```python
from build123d import *

# Parameters (mm, degrees)
SKETCH1_W           = 311.15
SKETCH1_H           = 266.7
SKETCH1_W_2         = 295.275
SKETCH1_H_2         = 250.825
BOSS_EXTRUDE1_DEPTH = 20.6375
SKETCH2_R           = 2.54
CUT_EXTRUDE1_DEPTH  = 320.049014669
SKETCH3_R           = 2.54
CUT_EXTRUDE2_DEPTH  = 373.362542974


with BuildPart() as part:
    # Sketch1 → Boss-Extrude1 (new body)
    with BuildSketch(Plane(origin=(0, 0, 0), x_dir=(1, 0, 0), z_dir=(0, 1, 0))):
        with Locations((-18.31426751, -70.1534017)):
            Rectangle(SKETCH1_W, SKETCH1_H)
        with Locations((-18.31426751, -70.1534017)):
            Rectangle(SKETCH1_W_2, SKETCH1_H_2, mode=Mode.SUBTRACT)
    extrude(amount=BOSS_EXTRUDE1_DEPTH)

    # Sketch2 → Cut-Extrude1 (cut, through all)
    with BuildSketch(Plane.XY.offset(203.5034017)):
        with Locations((-18.31426751, 10.31875)):
            Circle(SKETCH2_R)
    extrude(amount=-CUT_EXTRUDE1_DEPTH, mode=Mode.SUBTRACT)

    # Sketch3 → Cut-Extrude2 (cut, through all)
    with BuildSketch(Plane(origin=(137.26073249, 0, 0), x_dir=(0, 0, -1), z_dir=(1, 0, 0))):
        with Locations((-70.1534017, 10.31875)):
            Circle(SKETCH3_R)
    extrude(amount=-CUT_EXTRUDE2_DEPTH, mode=Mode.SUBTRACT)


solid = part.part
```
Verification items for the finished model (mm, model axes). A direction names the side the tool comes from. Give positions to 0.01 mm unless a question says otherwise; leave off trailing zeros. Order: outer loops, then holes, each group sorted by start corner. A loop starts at its lowest first (then second) coordinate and runs counter-clockwise, first axis right, second up. Notation, with made-up numbers: (49, 15.25) -> (96, 15.25) arc R36 ccw to (96, 49.25) -> close; hole circle Ø2 at (69, 33). An arc over 180 degrees is marked (long way). Use a Markdown table: item, result.
1) Section check B-B, the plane z = 181.5. Record the boundary of the cut face in (x, y), then the cut area to 3 significant figures.
Results:
| item | result |
|---|---|
| outline | (-173.89, 0) -> (-165.95, 0) -> (-165.95, 20.64) -> (-173.89, 20.64) -> close; (129.32, 0) -> (137.26, 0) -> (137.26, 20.64) -> (129.32, 20.64) -> close |
| area | 328 mm² |
2) Section check A-A, the plane x = -72. Record the boundary of the cut face in (y, z), then the cut area to 3 significant figures.
Results:
| item | result |
|---|---|
| outline | (0, -63.2) -> (20.64, -63.2) -> (20.64, -55.26) -> (0, -55.26) -> close; (0, 195.57) -> (20.64, 195.57) -> (20.64, 203.5) -> (0, 203.5) -> close |
| area | 328 mm² |
3) Material ranges on probe 1 along X at (y, z) = (4.75, 80); probe 2 along Z at (x, y) = (-9.5, 5.75), recorded low to high.
Results:
| item | result |
|---|---|
| probe 1 | -173.89 to -165.95, 129.32 to 137.26 |
| probe 2 | -63.2 to -55.26, 195.57 to 203.5 |
4) Mould release check, pull along X, two halves, no side actions. Record for faces 1 (the flat face through (-165.952, 12.5, 71.9)), 2 (the flat face through (-20.5, 12.5, 203.503)), 3 (the flat face through (137.261, 12.5, 72)): pulls with the +X half, pulls with the -X half, needs draft (parallel to the pull), parting line crosses it, or undercut.
Results:
| item | result |
|---|---|
| face 1 | undercut |
| face 2 | needs draft |
| face 3 | pulls with the +X half |
5) Tool access check on faces 4 (the flat face through (-20.4, 12.5, 195.566)), 5 (the flat face through (-31, 20.638, 198)). Record the directions out of +Z, -Z, +X, -X, +Y, -Y that give a thin tool (end or side, any length) a straight path to the whole face; none if there is none.
Results:
| item | result |
|---|---|
| face 4 | +Y, -Y |
| face 5 | +Z, -Z, +X, -X, +Y |
6) Depth check by flat-ended pin: pin 1 Ø4 at (y, z) = (10.32, 70.15) entering from +X. Enter the tip coordinate at first touch or a pass-through.
Results:
| item | result |
|---|---|
| pin 1 | through |
